Source: CAD feature listing. Evaluate the final solid. Frame: model axes, mm. A direction names the side the tool comes from. Coordinates: 2 decimals unless noted, no trailing zeros. Order: outer loops, then holes, each group sorted by start corner. A loop starts at its lowest first (then second) coordinate and runs counter-clockwise, first axis right, second up.
Item 1: Section B-B on y = 4.5. Return the cut outline in (x, z).
Item 2: Ray query, line 1 (X direction, y = 3.25, z = 38.5); line 2 (X direction, y = 1.5, z = 48); line 3 (Y direction, x = 5.5, z = 44). Return the intervals inside material, ascending.
Item 3: Contact query for flat-ended pins moving along their axis: P1, Ø1.9, axis at x = 12.5, z = 48, coming from the +Y side; P2, Ø5.5, axis at x = 12.5, z = 43, coming from the +Y side. Output: stop coordinate, or through.
Item 4: Section C-C on z = 42.75. Return the cut outline in (x, y).
Item 5: Reachability of faces 1 (the flat face through (3.3, 4, 41)), 2 (the flat face through (0, 3, 41)) from +Z, -Z, +X, -X, +Y, -Y: full face, straight path, thin tool, end or side. Return the list, or none.
Item 6: Mould query, pull axis Z, two halves, no side actions, for faces 3 (the flat face through (21.7, 4, 40)), 4 (the cylindrical face through (12.702, 3.521, 57.198)), 5 (the flat face through (12, 1, 33)), 6 (the flat face through (13, 0, 44)). Classes: released by +Z, released by -Z, zero draft, split by the parting line, or undercut.
from build123d import *

# Parameters (mm, degrees)
SKETCH_1_R           = 2.55
SKETCH_1_R_2         = 7.5
EXTRUDE_1_DEPTH      = 5
FILLET_2_R           = 5
CUT_EXTRUDE_1_DEPTH  = 109.559891304
EXTRUDE_2_DEPTH      = 5
SKETCH_3_R           = 1.55
CUT_EXTRUDE_2_DEPTH  = 109.559891304
FILLET_3_R           = 2
SKETCH_5_R           = 3
CUT_EXTRUDE_3_DEPTH  = 3
SKETCH_6_OUTSIDE_W   = 117.274
SKETCH_6_OUTSIDE_H   = 115.837
SKETCH_6_OUTSIDE_W_2 = 25
SKETCH_6_OUTSIDE_H_2 = 29.920384019
CUT_EXTRUDE_4_DEPTH  = 109.559891304
EXTRUDE_START        = -2
SKETCH_7_R           = 1.55
EXTRUDE_3_DEPTH      = 2
SKETCH_8_W           = 18.4
SKETCH_8_H           = 0.01
EXTRUDE_4_DEPTH      = 3


with BuildPart() as part:
    # ｽｹｯﾁ1 → ﾎﾞｽ - 押し出し1 (new body)
    with BuildSketch(Plane(origin=(0, 0, 0), x_dir=(1, 0, 0), z_dir=(0, 1, 0))):
        with BuildLine():
            Line((0, 0), (0, -48))
            ThreePointArc((0, -48), (12.5, -60.5), (25, -48))
            Line((25, -48), (25, -20))
            Line((25, -20), (90, -20))
            Line((90, -20), (90, 30))
            Line((90, 30), (0, 0))
        make_face()
        with Locations(Location((75.769750529, 14.715657976, 0), (0, 0, 270))):
            Circle(SKETCH_1_R, mode=Mode.SUBTRACT)
        with Locations(Location((75, -10, 0), (0, 0, 270))):
            Circle(SKETCH_1_R, mode=Mode.SUBTRACT)
        with Locations(Location((25, -10, 0), (0, 0, 270))):
            Circle(SKETCH_1_R, mode=Mode.SUBTRACT)
        with Locations(Location((12.5, -48, 0), (0, 0, 270))):
            Circle(SKETCH_1_R_2, mode=Mode.SUBTRACT)
    extrude(amount=EXTRUDE_1_DEPTH)

    # ﾌｨﾚｯﾄ2
    fillet_2_edges = [part.edges().sort_by_distance(p)[0] for p in [
        (90, 2.5, -30),
        (90, 2.5, 20),
    ]]
    fillet(fillet_2_edges, radius=FILLET_2_R)

    # ｽｹｯﾁ2 → ｶｯﾄ - 押し出し1 (cut, through all)
    with BuildSketch(Plane(origin=(0, 5, 0), x_dir=(1, 0, 0), z_dir=(0, 1, 0))):
        with BuildLine():
            Line((3.3, -48), (3.3, -33))
            Line((3.3, -33), (21.7, -33))
            Line((21.7, -33), (21.7, -48))
            ThreePointArc((21.7, -48), (12.5, -57.2), (3.3, -48))
        make_face()
    extrude(amount=-CUT_EXTRUDE_1_DEPTH, mode=Mode.SUBTRACT)

    # ｽｹｯﾁ4 → ﾎﾞｽ - 押し出し2 (add)
    with BuildSketch(Plane(origin=(0, 5, 0), x_dir=(1, 0, 0), z_dir=(0, 1, 0))):
        Polygon((0, 0), (0, 20), (60, 20), align=None)
    extrude(amount=-EXTRUDE_2_DEPTH)

    # ｽｹｯﾁ3 → ｶｯﾄ - 押し出し2 (cut, through all)
    with BuildSketch(Plane(origin=(0, 5, 0), x_dir=(1, 0, 0), z_dir=(0, 1, 0))):
        with Locations(Location((20.5, 5, 0), (0, 0, 270))):
            Circle(SKETCH_3_R)
        with Locations(Location((4.5, 5, 0), (0, 0, 90))):
            Circle(SKETCH_3_R)
    extrude(amount=-CUT_EXTRUDE_2_DEPTH, mode=Mode.SUBTRACT)

    # ﾌｨﾚｯﾄ3
    fillet_3_edges = [part.edges().sort_by_distance(p)[0] for p in [
        (60, 2.5, -20),
        (0, 2.5, -20),
    ]]
    fillet(fillet_3_edges, radius=FILLET_3_R)

    # ｽｹｯﾁ5 → ｶｯﾄ - 押し出し3 (cut)
    with BuildSketch(Plane.XZ.offset(-5)):
        with Locations(Location((4.5, -5, 0), (0, 0, 270))):
            Circle(SKETCH_5_R)
        with Locations(Location((20.5, -5, 0), (0, 0, 270))):
            Circle(SKETCH_5_R)
    extrude(amount=CUT_EXTRUDE_3_DEPTH, mode=Mode.SUBTRACT)

    # ｽｹｯﾁ6 outside → ｶｯﾄ - 押し出し4 (cut, through all)
    with BuildSketch(Plane(origin=(0, 5, 0), x_dir=(1, 0, 0), z_dir=(0, 1, 0))):
        with Locations((45, -16.2185)):
            Rectangle(SKETCH_6_OUTSIDE_W, SKETCH_6_OUTSIDE_H)
        with Locations((12.5, -47.96019201)):
            Rectangle(SKETCH_6_OUTSIDE_W_2, SKETCH_6_OUTSIDE_H_2, mode=Mode.SUBTRACT)
    extrude(amount=-CUT_EXTRUDE_4_DEPTH, mode=Mode.SUBTRACT)

    # ｽｹｯﾁ7 → ﾎﾞｽ - 押し出し3 (add)
    with BuildSketch(Plane.XZ.offset(EXTRUDE_START)):
        with BuildLine():
            Line((3.3, 33), (3.3, 48))
            ThreePointArc((3.3, 48), (12.5, 57.2), (21.7, 48))
            Line((21.7, 48), (21.7, 33))
            Line((21.7, 33), (3.3, 33))
        make_face()
        with Locations(Location((12.5, 48, 0), (0, 0, 270))):
            Circle(SKETCH_7_R, mode=Mode.SUBTRACT)
    extrude(amount=EXTRUDE_3_DEPTH)

    # ｽｹｯﾁ8 → ﾎﾞｽ - 押し出し4 (add)
    with BuildSketch(Plane(origin=(0, 2, 0), x_dir=(1, 0, 0), z_dir=(0, 1, 0))):
        with Locations((12.5, -33.005)):
            Rectangle(SKETCH_8_W, SKETCH_8_H)
    extrude(amount=EXTRUDE_4_DEPTH)


solid = part.part
Answer list:
1. outline: (0, 33) - (25, 33) - (25, 48) arc R12.5 ccw to (0, 48) - close; hole (3.3, 33.01) - (21.7, 33.01) - (21.7, 48) arc R9.2 ccw to (3.3, 48) - close
2. line 1: x = 0 to 3.3, 21.7 to 25
2. line 2: x = 0 to 10.95, 14.05 to 25
2. line 3: y = 0 to 2
3. P1: passes through
3. P2: stops at y = 2
4. outline: (0, 0) - (25, 0) - (25, 5) - (21.7, 5) - (21.7, 2) - (3.3, 2) - (3.3, 5) - (0, 5) - close
5. face 1: +Y
5. face 2: +Z, -Z, -X, +Y, -Y
6. face 3: undercut
6. face 4: undercut
6. face 5: released by -Z
6. face 6: zero draft
